Read the model definition and answer for the solid it produces. Units are mm, in the model's axes. A direction names the side the tool comes from. Coordinates: 2 decimals unless noted, no trailing zeros. Order: outer loops, then holes, each group sorted by start corner. A loop starts at its lowest first (then second) coordinate and runs counter-clockwise, first axis right, second up.
from build123d import *

# Parameters (mm, degrees)
EXTRUDE1_DEPTH = 6.35
SKETCH2_R      = 1.3335
EXTRUDE2_DEPTH = 4.572
SKETCH3_R      = 1.3335
EXTRUDE3_DEPTH = 5.08


with BuildPart() as part:
    # Sketch1 → Extrude1 (new body)
    with BuildSketch(Plane.XY):
        Polygon((1.888017478, 3.056790202), (-1.70324923, 3.163466199), (-3.591266708, 0.106675997), (-1.888017478, -3.056790202), (1.70324923, -3.163466199), (3.591266708, -0.106675997), align=None)
    extrude(amount=EXTRUDE1_DEPTH)

    # Sketch2 → Extrude2 (add)
    with BuildSketch(Plane.XY.offset(6.35)):
        Circle(SKETCH2_R)
    extrude(amount=EXTRUDE2_DEPTH)

    # Sketch3 → Extrude3 (cut)
    with BuildSketch(Plane(origin=(0, 0, 0), x_dir=(-1, 0, 0), z_dir=(0, 0, -1))):
        with Locations(Location((0, 0, 0), (0, 0, 180))):
            Circle(SKETCH3_R)
    extrude(amount=-EXTRUDE3_DEPTH, mode=Mode.SUBTRACT)


solid = part.part
Q1. The part is cut by section C-C, the plane x = -0.5. Determine the outline of the cut face in (y, z).
Q2. Determine the mould class of faces 3 (the cylindrical face through (0.62, 1.18, 2.5)), 4 (the flat face through (-2.752, -1.453, 3.131)), 5 (the flat face through (0, 0, 5.08)), 6 (the cylindrical face through (0.62, -1.18, 8.6)) for opening direction X: +X half, -X half, draft (parallel to the pull), parting line (faces both ways), or undercut.
Q3. Each of these flat-tipped pins is pushed along its axis until it touches: P1, Ø0.8, axis at x = 0.5, y = 0, coming from the -Z side; P2, Ø2, axis at x = -1.5, z = 5.5, coming from the +Y side; P3, Ø1.5, axis at y = -0.5, z = 2, coming from the -X side; P4, Ø2, axis at x = 0, z = 9, coming from the -Y side. Where does it stop, or does it pass through?
Q4. Straight lines are drawn through the part: L1, parallel to Y at x = 0, z = 3.6; L2, parallel to Z at x = 2, y = -2.25; L3, parallel to Y at x = 0.75, z = 4.5. For each, find the intervals that lie inside material, in ascending order.
Q5. The part is cut by section D-D, the plane z = 9. Determine the outline of the cut face in (x, y).
Q6. The part is cut by section A-A, the plane z = 2. Determine the outline of the cut face in (x, y), then the cut area to 3 significant figures.
Q7. The part is cut by section B-B, the plane y = -0.5. Determine the outline of the cut face in (x, z), then the cut area to 3 significant figures.
Q8. Which of the six approach directions +Z, -Z, +X, -X, +Y, -Y give full straight-line access (tool end or side, diameter ignored) to faces 1 (the flat face through (-0.1, 1.5, 6.35)), 2 (the flat face through (2.63, -1.66, 3.13))?
Computed values:
1. outline: (-3.1, 0) - (-1.24, 0) - (-1.24, 5.08) - (1.24, 5.08) - (1.24, 0) - (3.13, 0) - (3.13, 6.35) - (1.24, 6.35) - (1.24, 10.92) - (-1.24, 10.92) - (-1.24, 6.35) - (-3.1, 6.35) - close
2. face 3: undercut
2. face 4: -X half
2. face 5: undercut
2. face 6: parting line
3. P1: stops at z = 5.08
3. P2: stops at y = 3.16
3. P3: stops at x = -3.59
3. P4: stops at y = -1.33
4. L1: y = -3.11 to -1.33, 1.33 to 3.11
4. L2: z = 0 to 6.35
4. L3: y = -3.14 to -1.1, 1.1 to 3.09
5. outline: circle Ø2.67 at (0, 0)
6. outline: (-3.59, 0.11) - (-1.89, -3.06) - (1.7, -3.16) - (3.59, -0.11) - (1.89, 3.06) - (-1.7, 3.16) - close; hole circle Ø2.67 at (0, 0)
6. area: 28.0 mm2
7. outline: (-3.26, 0) - (-1.24, 0) - (-1.24, 5.08) - (1.24, 5.08) - (1.24, 0) - (3.35, 0) - (3.35, 6.35) - (1.24, 6.35) - (1.24, 10.92) - (-1.24, 10.92) - (-1.24, 6.35) - (-3.26, 6.35) - close
7. area: 40.7 mm2
8. face 1: +Z
8. face 2: +Z, -Z, +X, -Y
